CAD build for the part. Positions are in the model's coordinates, mm. Face numbers are marked on the shaded views. A direction names the side the tool comes from. Give positions to 0.01 mm unless a question says otherwise; leave off trailing zeros. Loops run counter-clockwise (first coordinate to the right, second up) from the corner with the lowest first, then second, coordinate; pieces in that order, holes last. Notation, with made-up numbers: (30.25, 64) -> (61.25, 64) arc R21 ccw to (61.25, 101) -> close; hole circle Ø11 at (-33.75, 73.25). An arc over 180 degrees is marked (long way). Use one line per item in the form item = value.
```python
from build123d import *

# Parameters (mm, degrees)
SKETCH1_R                      = 2
BASE_FLANGE1_DEPTH             = 1.6
EDGE_FLANGE1_STRIP_W           = 8.4
EDGE_FLANGE1_STRIP_H           = 1.6
EDGE_FLANGE1_STRIP_CUT_DEPTH   = 8
EDGE_FLANGE1_STRIP_2_W         = 8.4
EDGE_FLANGE1_STRIP_2_H         = 1.6
EDGE_FLANGE1_STRIP_CUT_2_DEPTH = 8
EDGE_FLANGE1_STRIP_3_W         = 8.4
EDGE_FLANGE1_STRIP_3_H         = 1.6
EDGE_FLANGE1_STRIP_CUT_3_DEPTH = 42
EDGE_FLANGE1_DEPTH             = 8
EDGE_FLANGE1_BEND_DEPTH        = 8
EDGE_FLANGE1_BEND_2_DEPTH      = 42
CUT_EXTRUDE1_REACH             = 54.532
SKETCH14_R                     = 3
CUT_EXTRUDE2_REACH             = 51.136
SKETCH15_R                     = 2


# Sheet-metal steps are written as plain solids
with BuildPart() as part:
    # Sketch1 → Base-Flange1 (new body)
    with BuildSketch(Plane(origin=(0, 0, 0), x_dir=(1, 0, 0), z_dir=(0, 1, 0))):
        Polygon((-18.514, 21), (-13.514, 21), (-13.514, 29), (13.514, 29), (13.514, 21), (9.514, 21), (9.514, 18), (18.514, 18), (18.514, -18), (9.514, -18), (9.514, -21), (13.514, -21), (13.514, -29), (-13.514, -29), (-13.514, -21), (-18.514, -21), align=None)
        with Locations(Location((-6.514, 26, 0), (0, 0, 270))):
            Circle(SKETCH1_R, mode=Mode.SUBTRACT)
        with Locations(Location((6.514, 26, 0), (0, 0, 270))):
            Circle(SKETCH1_R, mode=Mode.SUBTRACT)
        with Locations(Location((6.514, -26, 0), (0, 0, 90))):
            Circle(SKETCH1_R, mode=Mode.SUBTRACT)
        with Locations(Location((-6.514, -26, 0), (0, 0, 90))):
            Circle(SKETCH1_R, mode=Mode.SUBTRACT)
    extrude(amount=-BASE_FLANGE1_DEPTH)

    # Edge-Flange1 strip (across the edge) → Edge-Flange1 strip cut (cut)
    with BuildSketch(Plane(origin=(13.514, 0, 29), x_dir=(-1, 0, 0), z_dir=(0, 0, -1))):
        with Locations((-1.6, -0.8)):
            Rectangle(EDGE_FLANGE1_STRIP_W, EDGE_FLANGE1_STRIP_H)
    extrude(amount=EDGE_FLANGE1_STRIP_CUT_DEPTH, mode=Mode.SUBTRACT)

    # Edge-Flange1 strip 2 (across the edge) → Edge-Flange1 strip cut 2 (cut)
    with BuildSketch(Plane(origin=(13.514, 0, -21), x_dir=(-1, 0, 0), z_dir=(0, 0, -1))):
        with Locations((-1.6, -0.8)):
            Rectangle(EDGE_FLANGE1_STRIP_2_W, EDGE_FLANGE1_STRIP_2_H)
    extrude(amount=EDGE_FLANGE1_STRIP_CUT_2_DEPTH, mode=Mode.SUBTRACT)

    # Edge-Flange1 strip 3 (across the edge) → Edge-Flange1 strip cut 3 (cut)
    with BuildSketch(Plane(origin=(-18.514, 0, -21), x_dir=(1, 0, 0), z_dir=(0, 0, 1))):
        with Locations((-1.6, -0.8)):
            Rectangle(EDGE_FLANGE1_STRIP_3_W, EDGE_FLANGE1_STRIP_3_H)
    extrude(amount=EDGE_FLANGE1_STRIP_CUT_3_DEPTH, mode=Mode.SUBTRACT)

    # Edge-Flange1 section (across the edge) → Edge-Flange1 (add)
    with BuildSketch(Plane(origin=(13.514, 0, 29), x_dir=(-1, 0, 0), z_dir=(0, 0, -1))):
        with BuildLine():
            Line((0, 1), (0, 23.4))
            Line((0, 23.4), (1.6, 23.4))
            Line((1.6, 23.4), (1.6, 1))
            ThreePointArc((1.6, 1), (1.892893219, 0.292893219), (2.6, 0))
            Line((2.6, 0), (2.6, -1.6))
            ThreePointArc((2.6, -1.6), (0.761522369, -0.838477631), (0, 1))
        make_face()
    extrude(amount=EDGE_FLANGE1_DEPTH)

    # Edge-Flange1 section 2 (across the edge) → Edge-Flange1 bend (add)
    with BuildSketch(Plane(origin=(13.514, 0, -21), x_dir=(-1, 0, 0), z_dir=(0, 0, -1))):
        with BuildLine():
            Line((0, 1), (0, 23.4))
            Line((0, 23.4), (1.6, 23.4))
            Line((1.6, 23.4), (1.6, 1))
            ThreePointArc((1.6, 1), (1.892893219, 0.292893219), (2.6, 0))
            Line((2.6, 0), (2.6, -1.6))
            ThreePointArc((2.6, -1.6), (0.761522369, -0.838477631), (0, 1))
        make_face()
    extrude(amount=EDGE_FLANGE1_BEND_DEPTH)

    # Edge-Flange1 section 3 (across the edge) → Edge-Flange1 bend 2 (add)
    with BuildSketch(Plane(origin=(-18.514, 0, -21), x_dir=(1, 0, 0), z_dir=(0, 0, 1))):
        with BuildLine():
            Line((0, 1), (0, 23.4))
            Line((0, 23.4), (1.6, 23.4))
            Line((1.6, 23.4), (1.6, 1))
            ThreePointArc((1.6, 1), (1.892893219, 0.292893219), (2.6, 0))
            Line((2.6, 0), (2.6, -1.6))
            ThreePointArc((2.6, -1.6), (0.761522369, -0.838477631), (0, 1))
        make_face()
    extrude(amount=EDGE_FLANGE1_BEND_2_DEPTH)

    # Sketch14 → Cut-Extrude1 (cut, up to next)
    with BuildSketch(Plane.ZY.offset(18.514), mode=Mode.PRIVATE) as cut_extrude1_sk1:
        with Locations(Location((0, 11.045309813, 0), (0, 0, 270))):
            Circle(SKETCH14_R)
    cut_extrude1_tool1 = extrude(cut_extrude1_sk1.sketch, amount=-CUT_EXTRUDE1_REACH, mode=Mode.PRIVATE) & part.part
    add(cut_extrude1_tool1.solids().sort_by_distance((-18.514, 11.04531, 0))[0], mode=Mode.SUBTRACT)

    # Sketch15 → Cut-Extrude2 (cut, up to next)
    with BuildSketch(Plane(origin=(13.514, 0, 0), x_dir=(0, 0, -1), z_dir=(1, 0, 0)), mode=Mode.PRIVATE) as cut_extrude2_sk1:
        with Locations(Location((-24.13, 7, 0), (0, 0, 90))):
            Circle(SKETCH15_R)
    cut_extrude2_tool1 = extrude(cut_extrude2_sk1.sketch, amount=-CUT_EXTRUDE2_REACH, mode=Mode.PRIVATE) & part.part
    # Sketch15 → Cut-Extrude2 (cut, up to next)
    with BuildSketch(Plane(origin=(13.514, 0, 0), x_dir=(0, 0, -1), z_dir=(1, 0, 0)), mode=Mode.PRIVATE) as cut_extrude2_sk2:
        with Locations(Location((-24.13, 17.16, 0), (0, 0, 90))):
            Circle(SKETCH15_R)
    cut_extrude2_tool2 = extrude(cut_extrude2_sk2.sketch, amount=-CUT_EXTRUDE2_REACH, mode=Mode.PRIVATE) & part.part
    # Sketch15 → Cut-Extrude2 (cut, up to next)
    with BuildSketch(Plane(origin=(13.514, 0, 0), x_dir=(0, 0, -1), z_dir=(1, 0, 0)), mode=Mode.PRIVATE) as cut_extrude2_sk3:
        with Locations(Location((24.13, 7, 0), (0, 0, 270))):
            Circle(SKETCH15_R)
    cut_extrude2_tool3 = extrude(cut_extrude2_sk3.sketch, amount=-CUT_EXTRUDE2_REACH, mode=Mode.PRIVATE) & part.part
    # Sketch15 → Cut-Extrude2 (cut, up to next)
    with BuildSketch(Plane(origin=(13.514, 0, 0), x_dir=(0, 0, -1), z_dir=(1, 0, 0)), mode=Mode.PRIVATE) as cut_extrude2_sk4:
        with Locations(Location((24.13, 17.16, 0), (0, 0, 270))):
            Circle(SKETCH15_R)
    cut_extrude2_tool4 = extrude(cut_extrude2_sk4.sketch, amount=-CUT_EXTRUDE2_REACH, mode=Mode.PRIVATE) & part.part
    add(cut_extrude2_tool1.solids().sort_by_distance((13.514, 7, 24.13))[0], mode=Mode.SUBTRACT)
    add(cut_extrude2_tool2.solids().sort_by_distance((13.514, 17.16, 24.13))[0], mode=Mode.SUBTRACT)
    add(cut_extrude2_tool3.solids().sort_by_distance((13.514, 7, -24.13))[0], mode=Mode.SUBTRACT)
    add(cut_extrude2_tool4.solids().sort_by_distance((13.514, 17.16, -24.13))[0], mode=Mode.SUBTRACT)


solid = part.part
```
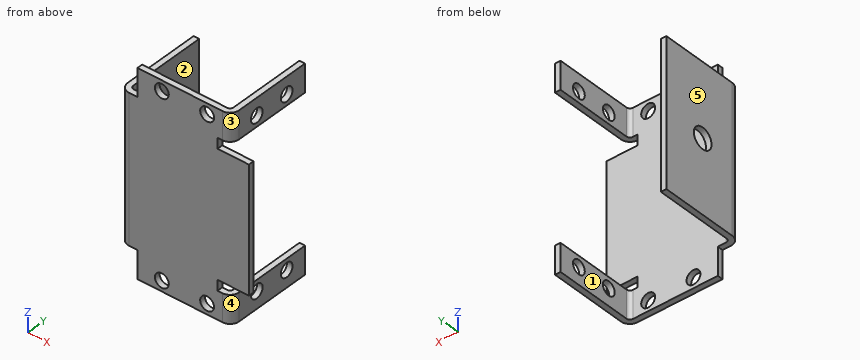
1. Drill centre lines: line 1 (Z direction, x = 13.1, y = 17.16); line 2 (X direction, y = 9, z = 2.5); line 3 (Y direction, x = -4, z = -3). Where is each one in solid material? Low to high.
Result sheet:
line_1 = -29 to -26.13, -22.13 to -21, 21 to 22.13, 26.13 to 29
line_2 = -18.51 to -16.91
line_3 = -1.6 to 0
2. Cut at A-A, the plane y = 4.25. Write the cut outline in (x, z), then the cut area to 3 significant figures.
Result sheet:
outline = (-18.51, -21) -> (-16.91, -21) -> (-16.91, 21) -> (-18.51, 21) -> close; (11.91, -29) -> (13.51, -29) -> (13.51, -21) -> (11.91, -21) -> close; (11.91, 21) -> (13.51, 21) -> (13.51, 29) -> (11.91, 29) -> close
area = 92.8 mm^2
3. Tool access for the marked faces 1, 2, 3, 4 and 5: list every direction of +Z, -Z, +X, -X, +Y, -Y with a clear straight run to the whole face (end or side of a thin tool).
Result sheet:
face_1 = +Z, -Z, -X, +Y
face_2 = +Z, -Z, +X, +Y
face_3 = +Z, +X, -Y
face_4 = -Z, +X, -Y
face_5 = +Z, -Z, -X, +Y, -Y
4. Drop flat-ended pins along their axis: P1, Ø11, axis at y = 15, z = -9, coming from the +X side; P2, Ø6.5, axis at y = 12, z = 25.5, coming from the -X side; P3, Ø1.3, axis at x = 16, y = -1, coming from the -Z side; P4, Ø8, axis at x = 11.5, z = -22, coming from the -Y side. Give the stop position or say it passes through.
Result sheet:
P1 = -16.91
P2 = 11.91
P3 = -18
P4 = -1.6
5. Cut at B-B, the plane z = 0. Write the cut outline in (x, y).
Result sheet:
outline = (-18.51, 1) arc R2.6 ccw to (-15.91, -1.6) -> (18.51, -1.6) -> (18.51, 0) -> (-15.91, 0) arc R1 cw to (-16.91, 1) -> (-16.91, 8.05) -> (-18.51, 8.05) -> close; (-18.51, 14.05) -> (-16.91, 14.05) -> (-16.91, 23.4) -> (-18.51, 23.4) -> close
6. Cut at C-C, the plane y = 7. Write the cut outline in (x, z), then the cut area to 3 significant figures.
Result sheet:
outline = (-18.51, -21) -> (-16.91, -21) -> (-16.91, 21) -> (-18.51, 21) -> close; (11.91, -29) -> (13.51, -29) -> (13.51, -26.13) -> (11.91, -26.13) -> close; (11.91, -22.13) -> (13.51, -22.13) -> (13.51, -21) -> (11.91, -21) -> close; (11.91, 21) -> (13.51, 21) -> (13.51, 22.13) -> (11.91, 22.13) -> close; (11.91, 26.13) -> (13.51, 26.13) -> (13.51, 29) -> (11.91, 29) -> close
area = 80.0 mm^2
7. Cut at D-D, the plane y = 16. Write the cut outline in (x, z).
Result sheet:
outline = (-18.51, -21) -> (-16.91, -21) -> (-16.91, 21) -> (-18.51, 21) -> close; (11.91, -29) -> (13.51, -29) -> (13.51, -25.76) -> (11.91, -25.76) -> close; (11.91, -22.5) -> (13.51, -22.5) -> (13.51, -21) -> (11.91, -21) -> close; (11.91, 21) -> (13.51, 21) -> (13.51, 22.5) -> (11.91, 22.5) -> close; (11.91, 25.76) -> (13.51, 25.76) -> (13.51, 29) -> (11.91, 29) -> close
